Here's how the part is built. I have some questions about the finished solid (model axes, mm). A direction names the side the tool comes from. Give positions to 0.01 mm unless a question says otherwise; leave off trailing zeros. Loops run counter-clockwise (first coordinate to the right, second up) from the corner with the lowest first, then second, coordinate; pieces in that order, holes last.
Q1. For faces 1 (the face through (0, 9, 1)), 2 (the face through (5.96, 1.88, 2.74)), which set-ups out of +Z, -Z, +X, -X, +Y, -Y let a thin tool reach every point of the face, with its end or its side?
Q2. Suppose I cut it at A-A (y = 0). List the corners of the cut face in (x, z) for me.
Q3. Thinking about a two-plate mould opening in X: for faces 3 (the face through (4.7, -4.7, 0)), 4 (the face through (-2.38, -10.74, 0.99)), 5 (the face through (-0.75, 5.7, 1.77)), which applies, pulls with the +X half, pulls with the -X half, needs draft (parallel to the pull), parting line crosses it, or undercut?
Q4. Suppose I cut it at C-C (y = -3). List the corners of the cut face in (x, z) for me, and give its area (3 significant figures).
Q5. Suppose I cut it at D-D (z = 2.4). List the corners of the cut face in (x, y) for me, and give its area (3 significant figures).
Q6. Suppose I cut it at B-B (x = 7.5). List the corners of the cut face in (y, z) for me.
Q7. I'm going to push flat-ended pins straight in: P1, Ø3, axis at x = -5.66, y = 5.66, coming from the -Z side; P2, Ø7, axis at x = 0, y = 0, coming from the -Z side (3 decimals); P3, Ø2, axis at y = -8.5, z = 2.5, coming from the -X side; P4, Ø2.5, axis at x = 8, y = 0, coming from the +Z side. Where does each tip first touch, or does it pass through?
Q8. I need wall thicknesses on probe 1 along Y at (x, z) = (0, 0.4); probe 2 along Y at (x, z) = (-4.75, 1); probe 3 along Z at (x, y) = (-2, 8.5). Which ranges of each line are inside material? Lowest first, please.
```python
from build123d import *

# Parameters (mm, degrees)
SKETCH1_R           = 11
SKETCH1_R_2         = 1
BOSS_EXTRUDE1_DEPTH = 2
SKETCH2_R           = 6.25
BOSS_EXTRUDE2_DEPTH = 1.5
SKETCH3_R           = 5.75
CUT_EXTRUDE1_DEPTH  = 11


with BuildPart() as part:
    # Sketch1 → Boss-Extrude1 (new body)
    with BuildSketch(Plane.XY):
        Circle(SKETCH1_R)
        with Locations((0, 8)):
            Circle(SKETCH1_R_2, mode=Mode.SUBTRACT)
        with Locations((5.656854249, 5.656854249)):
            Circle(SKETCH1_R_2, mode=Mode.SUBTRACT)
        with Locations((8, 0)):
            Circle(SKETCH1_R_2, mode=Mode.SUBTRACT)
        with Locations((5.656854249, -5.656854249)):
            Circle(SKETCH1_R_2, mode=Mode.SUBTRACT)
        with Locations((0, -8)):
            Circle(SKETCH1_R_2, mode=Mode.SUBTRACT)
        with Locations((-5.656854249, -5.656854249)):
            Circle(SKETCH1_R_2, mode=Mode.SUBTRACT)
        with Locations((-8, 0)):
            Circle(SKETCH1_R_2, mode=Mode.SUBTRACT)
        with Locations((-5.656854249, 5.656854249)):
            Circle(SKETCH1_R_2, mode=Mode.SUBTRACT)
    extrude(amount=BOSS_EXTRUDE1_DEPTH)

    # Sketch2 → Boss-Extrude2 (add)
    with BuildSketch(Plane.XY.offset(2)):
        Circle(SKETCH2_R)
    extrude(amount=BOSS_EXTRUDE2_DEPTH)

    # Sketch3 → Cut-Extrude1 (cut)
    with BuildSketch(Plane.XY.offset(3.5)):
        Circle(SKETCH3_R)
    extrude(amount=-CUT_EXTRUDE1_DEPTH, mode=Mode.SUBTRACT)


solid = part.part
```
Solutions:
1. face 1: +Z, -Z
1. face 2: +Z
2. outline: (-11, 0) - (-9, 0) - (-9, 2) - (-11, 2) - close; (-7, 0) - (-5.75, 0) - (-5.75, 3.5) - (-6.25, 3.5) - (-6.25, 2) - (-7, 2) - close; (5.75, 0) - (7, 0) - (7, 2) - (6.25, 2) - (6.25, 3.5) - (5.75, 3.5) - close; (9, 0) - (11, 0) - (11, 2) - (9, 2) - close
3. face 3: needs draft
3. face 4: parting line crosses it
3. face 5: undercut
4. outline: (-10.58, 0) - (-4.91, 0) - (-4.91, 3.5) - (-5.48, 3.5) - (-5.48, 2) - (-10.58, 2) - close; (4.91, 0) - (10.58, 0) - (10.58, 2) - (5.48, 2) - (5.48, 3.5) - (4.91, 3.5) - close
4. area: 24.4 mm2
5. outline: circle Ø12.5 at (0, 0); hole circle Ø11.5 at (0, 0)
5. area: 18.8 mm2
6. outline: (-8.05, 0) - (-0.87, 0) - (-0.87, 2) - (-8.05, 2) - close; (0.87, 0) - (8.05, 0) - (8.05, 2) - (0.87, 2) - close
7. P1: stops at z = 0
7. P2: passes through
7. P3: stops at x = -7.92
7. P4: stops at z = 2
8. probe 1: y = -11 to -9, -7 to -5.75, 5.75 to 7, 9 to 11
8. probe 2: y = -9.92 to -6.08, -5.24 to -3.24, 3.24 to 5.24, 6.08 to 9.92
8. probe 3: z = 0 to 2
